Check sheet for the drawn part. Datum: minimum x, y, z corner. Units: mm. A direction names the side the tool comes from. Give positions to 0.01 mm unless a question says otherwise; leave off trailing zeros. Order: outer loops, then holes, each group sorted by start corner. A loop starts at its lowest first (then second) coordinate and runs counter-clockwise, first axis right, second up. Notation, with made-up numbers: (35.5, 34) -> (73.5, 34) arc R4 cw to (73.5, 38) -> close; hole circle Ø10 at (18, -11). An arc over 180 degrees is marked (long way). Return JSON: item names as keys, results as strings. Group by question number.
(1) Cross-section at C-C on y = 16.5. Enter the section's corners in (x, z).
(2) Depth check by flat-ended pin: pin 1 Ø25 at (x, y) = (13.5, 34) entering from +Z; pin 2 Ø12 at (y, z) = (29, 91.5) entering from +X; pin 3 Ø1.5 at (y, z) = (51.5, 45.5) entering from +X. Enter the tip coordinate at first touch or a pass-through.
(3) Thickness scan on line 1 along X through (y, z) = (16.5, 50); line 2 along X through (y, z) = (32, 50); line 3 along Z through (x, y) = (81.5, 48.5). Record the ranges inside material, lowest first.
(4) Cross-section at B-B on x = 100. Enter the section's corners in (y, z), then the cut area to 4 significant figures.
(5) Tool access check on the marked faces 1, 2 and 3. Record the directions out of +Z, -Z, +X, -X, +Y, -Y that give a thin tool (end or side, any length) a straight path to the whole face; none if there is none.
(6) Cross-section at D-D on x = 60.5. Enter the section's corners in (y, z).
(7) Release check for a two-part mould opening along X. For the marked faces 4, 5 and 6 record: pulls with the +X half, pulls with the -X half, needs draft (parallel to the pull), parting line crosses it, or undercut.
(8) Cross-section at A-A on z = 50. Enter the section's corners in (x, y).
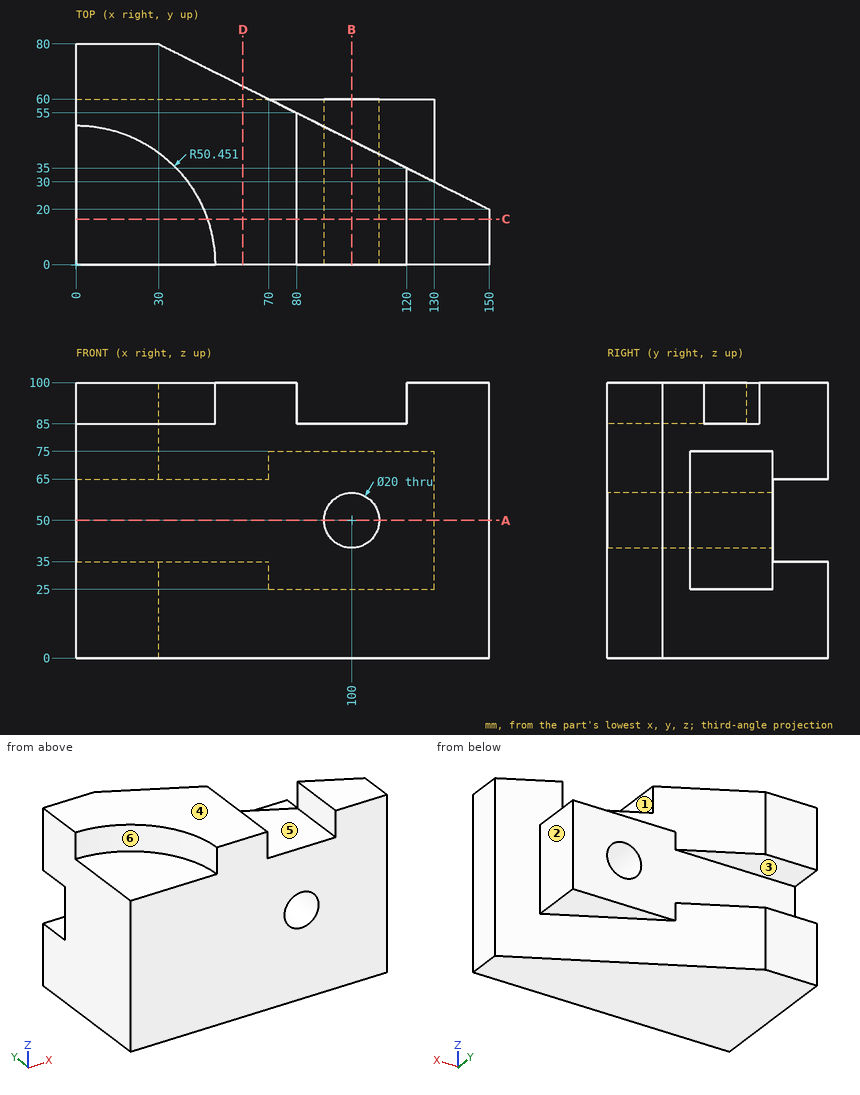
Verdict:
{
 "1": {"outline": "(0, 0) -> (150, 0) -> (150, 100) -> (120, 100) -> (120, 85) -> (80, 85) -> (80, 100) -> (47.68, 100) -> (47.68, 85) -> (0, 85) -> close; hole circle Ø20 at (100, 50)"},
 "2": {"pin 1": "z = 85", "pin 2": "x = 144", "pin 3": "x = 130"},
 "3": {"line 1": "0 to 90, 110 to 150", "line 2": "0 to 90, 110 to 130", "line 3": "0 to 85"},
 "4": {"outline": "(0, 0) -> (45, 0) -> (45, 25) -> (60, 25) -> (60, 40) -> (0, 40) -> close; (0, 60) -> (60, 60) -> (60, 75) -> (45, 75) -> (45, 85) -> (0, 85) -> close", "area": "3,375 mm²"},
 "5": {"face 1": "+Z, +Y, -Y", "face 2": "+Z, -Z, +X, +Y", "face 3": "+X, -X, +Y"},
 "6": {"outline": "(0, 0) -> (64.75, 0) -> (64.75, 35) -> (60, 35) -> (60, 65) -> (64.75, 65) -> (64.75, 100) -> (0, 100) -> close"},
 "7": {"face 4": "needs draft", "face 5": "undercut", "face 6": "pulls with the -X half"},
 "8": {"outline": "(0, 0) -> (90, 0) -> (90, 60) -> (0, 60) -> close; (110, 0) -> (150, 0) -> (150, 20) -> (130, 30) -> (130, 60) -> (110, 60) -> close"}
}
